```python
from build123d import *

# Parameters (mm, degrees)
F0_R     = 11.0109
F1_DEPTH = 7


with BuildPart() as f1:
    # F0 (on Top) → F1 (new body)
    with BuildSketch(Plane.XY):
        with BuildLine():
            Line((14.1859, 0), (11.0109, 0))
            ThreePointArc((11.0109, 0), (0, -11.0109), (-11.0109, 0))
            Line((-11.0109, 0), (-14.1859, 0))
            ThreePointArc((-14.1859, 0), (-4.0564627793, -13.5935598182), (11.8660062633, -7.7741658182))
            ThreePointArc((11.8660062633, -7.7741658182), (12.0777532722, -7.4348353952), (12.2853497755, -7.09295))
            ThreePointArc((12.2853497755, -7.09295), (12.4445825488, -6.7642227487), (12.6338376613, -6.4518140673))
            ThreePointArc((12.6338376613, -6.4518140673), (13.7924275689, -3.3179361907), (14.1859, 0))
        make_face()
        with BuildLine():
            ThreePointArc((-11.0109, 0), (0, 11.0109), (11.0109, 0))
            Line((11.0109, 0), (14.1859, 0))
            ThreePointArc((14.1859, 0), (4.0422659472, 13.5977882327), (-11.882216203, 7.7493675171))
            ThreePointArc((-11.882216203, 7.7493675171), (-12.0857093478, 7.4223418162), (-12.2853497755, 7.09295))
            ThreePointArc((-12.2853497755, 7.09295), (-12.4445825488, 6.7642227487), (-12.6338376613, 6.4518140673))
            ThreePointArc((-12.6338376613, 6.4518140673), (-13.7924275689, 3.3179361907), (-14.1859, 0))
            Line((-14.1859, 0), (-11.0109, 0))
        make_face()
        with BuildLine():
            Line((17.5641, 0), (14.1859, 0))
            ThreePointArc((14.1859, 0), (13.7924275689, -3.3179361907), (12.6338376613, -6.4518140673))
            ThreePointArc((12.6338376613, -6.4518140673), (15.875, -4.7244), (19.1161623387, -6.4518140673))
            ThreePointArc((19.1161623387, -6.4518140673), (17.9575724311, -3.3179361907), (17.5641, 0))
        make_face()
        with BuildLine():
            ThreePointArc((-11.882216203, 7.7493675171), (4.0422659472, 13.5977882327), (14.1859, 0))
            Line((14.1859, 0), (17.5641, 0))
            ThreePointArc((17.5641, 0), (27.7077340528, 13.5977882327), (43.632216203, 7.7493675171))
            ThreePointArc((43.632216203, 7.7493675171), (15.875, 23.0632), (-11.882216203, 7.7493675171))
        make_face()
        with BuildLine():
            Line((-17.5641, 0), (-14.1859, 0))
            ThreePointArc((-14.1859, 0), (-13.7924275689, 3.3179361907), (-12.6338376613, 6.4518140673))
            ThreePointArc((-12.6338376613, 6.4518140673), (-15.875, 4.7244), (-19.1161623387, 6.4518140673))
            ThreePointArc((-19.1161623387, 6.4518140673), (-17.9575724311, 3.3179361907), (-17.5641, 0))
        make_face()
        with BuildLine():
            ThreePointArc((11.8660062633, -7.7741658182), (-4.0564627793, -13.5935598182), (-14.1859, 0))
            Line((-14.1859, 0), (-17.5641, 0))
            ThreePointArc((-17.5641, 0), (-27.6935372207, -13.5935598182), (-43.6160062633, -7.7741658182))
            ThreePointArc((-43.6160062633, -7.7741658182), (-15.875, -23.0520875), (11.8660062633, -7.7741658182))
        make_face()
        with BuildLine():
            ThreePointArc((43.632216203, 7.7493675171), (27.7077340528, 13.5977882327), (17.5641, 0))
            ThreePointArc((17.5641, 0), (17.9575724311, -3.3179361907), (19.1161623387, -6.4518140673))
            ThreePointArc((19.1161623387, -6.4518140673), (19.3054174512, -6.7642227487), (19.4646502245, -7.09295))
            ThreePointArc((19.4646502245, -7.09295), (35.4215810919, -13.7025271792), (45.9359, 0))
            ThreePointArc((45.9359, 0), (45.4525271792, 3.6715810919), (44.0353497755, 7.09295))
            ThreePointArc((44.0353497755, 7.09295), (43.8357093478, 7.4223418162), (43.632216203, 7.7493675171))
        make_face()
        with BuildLine():
            ThreePointArc((42.7609, 0), (31.75, -11.0109), (20.7391, 0))
            ThreePointArc((20.7391, 0), (31.75, 11.0109), (42.7609, 0))
        make_face(mode=Mode.SUBTRACT)
        with BuildLine():
            ThreePointArc((-43.6160062633, -7.7741658182), (-27.6935372207, -13.5935598182), (-17.5641, 0))
            ThreePointArc((-17.5641, 0), (-17.9575724311, 3.3179361907), (-19.1161623387, 6.4518140673))
            ThreePointArc((-19.1161623387, 6.4518140673), (-19.3054174512, 6.7642227487), (-19.4646502245, 7.09295))
            ThreePointArc((-19.4646502245, 7.09295), (-38.84295, 12.2853497755), (-44.0353497755, -7.09295))
            ThreePointArc((-44.0353497755, -7.09295), (-43.8277532722, -7.4348353952), (-43.6160062633, -7.7741658182))
        make_face()
        with Locations((-31.75, 0)):
            Circle(F0_R, mode=Mode.SUBTRACT)
    extrude(amount=F1_DEPTH)


solid = f1.part
```
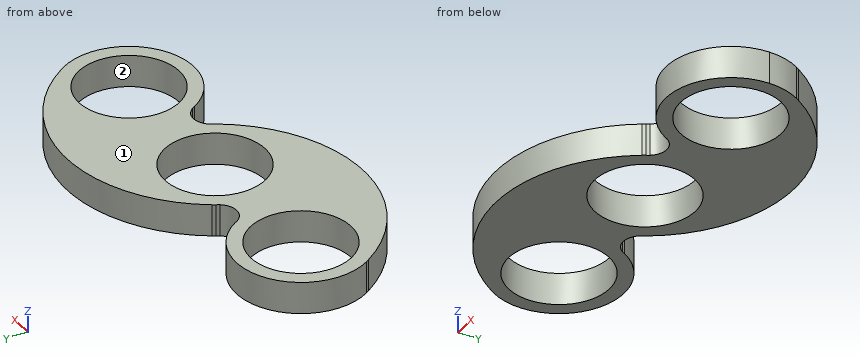
For this review, take the finished solid that the model builds, in its own axes (mm). Face numbers are marked on the shaded views. Give positions to 0.01 mm unless a question says otherwise; leave off trailing zeros. Write each loop counter-clockwise with the first axis right and the second up, starting at its lowest first coordinate (ties: lowest second). Pieces come first, ordered by that corner, then holes. Notation, with made-up numbers: M 31.5,-11 L 46.5,-11 A20 cw 46.5,5 Z; hole C -23,50 d9. An arc over 180 degrees is marked long. Answer as a JSON object with one key per item and string values. Group by question number.
Item 1: Consider section C-C on x = -31.75. Write out the cut boundary in (y, z).
Item 2: Draft analysis for pull direction X (two halves, no side actions). For the marked faces 1 and 2, state which applies: +X half, -X half, draft (parallel to the pull), parting line (faces both ways), or undercut.
Item 3: Consider section A-A on x = 1.5. Write out the cut boundary in (y, z), plus the area to 3 significant figures.
Item 4: For pin 1 Ø1.5 at (x, z) = (11, 3) entering from +Y; pin 2 Ø1.5 at (y, z) = (-13.5, 2) entering from -X; pin 3 Ø3 at (y, z) = (11.5, 3.5) entering from +X, all flat-tipped, find the tip position at first contact; note any pin that passes through.
Item 5: For probe 1 along X at (y, z) = (7.5, 4.5); probe 2 along X at (y, z) = (-6, 6.25); probe 3 along Y at (x, z) = (25.5, 5), list the stretches that pass through material, from the lowest coordinate up. Write a range as [from, to].
Item 6: Consider section B-B on z = 2.75. Count the separate pieces of the cut face and the enclosed holes in it, plus the area to 3 significant figures.
Item 7: Consider section D-D on x = 15.5. Write out the cut boundary in (y, z), plus the area to 3 significant figures.
Check result:
{
 "1": {"outline": "M -18.96,0 L -11.01,0 L -11.01,7 L -18.96,7 Z; M 11.01,0 L 14.19,0 L 14.19,7 L 11.01,7 Z"},
 "2": {"face 1": "draft", "face 2": "undercut"},
 "3": {"outline": "M -18.08,0 L -10.91,0 L -10.91,7 L -18.08,7 Z; M 10.91,0 L 19.75,0 L 19.75,7 L 10.91,7 Z", "area": "112 mm^2"},
 "4": {"pin 1": "stops at y = 22.8", "pin 2": "stops at x = -39.75", "pin 3": "stops at x = 42.08"},
 "5": {"probe 1": "x = [-43.79, -39.81], [-23.69, -19.71], [-12.04, -8.06], [8.06, 23.69], [39.81, 43.79]", "probe 2": "x = [-44.6, -40.98], [-22.52, -9.23], [9.23, 12.99], [18.76, 22.52], [40.98, 44.6]", "probe 3": "y = [-12.73, -9.07], [9.07, 21.62]"},
 "6": {"separate pieces": "1", "enclosed holes": "3", "area": "1,640 mm^2"},
 "7": {"outline": "M -4.74,0 L 23.06,0 L 23.06,7 L -4.74,7 Z", "area": "195 mm^2"}
}
